```python
from build123d import *

# Parameters (mm, degrees)
SKETCH_1_W          = 25
SKETCH_1_H          = 8
SKETCH_1_R          = 1.2
EXTRUDE_2_DEPTH     = 4
SKETCH_2_W          = 10
SKETCH_2_H          = 0.8
EXTRUDE_3_DEPTH     = 0.8
SKETCH_3_W          = 7.5
SKETCH_3_H          = 8
SKETCH_3_R          = 1.2
EXTRUDE_4_DEPTH     = 1.5
SKETCH_4_W          = 25
SKETCH_4_H          = 1
CUT_EXTRUDE_1_DEPTH = 19.5


with BuildPart() as part:
    # 草图1 → 凸台-拉伸2 (new body)
    with BuildSketch(Plane.XY):
        with Locations((0.109785312, -0.548926558)):
            Rectangle(SKETCH_1_W, SKETCH_1_H)
        with Locations((-8.390214688, -2.048926558)):
            Circle(SKETCH_1_R, mode=Mode.SUBTRACT)
        with Locations((8.609785312, -2.048926558)):
            Circle(SKETCH_1_R, mode=Mode.SUBTRACT)
    extrude(amount=EXTRUDE_2_DEPTH)

    # 草图2 → 凸台-拉伸3 (add)
    with BuildSketch(Plane.XY.offset(4)):
        with Locations((0.109785312, -3.748926558)):
            Rectangle(SKETCH_2_W, SKETCH_2_H)
        with Locations((0.109785312, -2.148926558)):
            Rectangle(SKETCH_2_W, SKETCH_2_H)
        with Locations((0.109785312, -0.548926558)):
            Rectangle(SKETCH_2_W, SKETCH_2_H)
        with Locations((0.109785312, 2.651073442)):
            Rectangle(SKETCH_2_W, SKETCH_2_H)
        with Locations((0.109785312, 1.051073442)):
            Rectangle(SKETCH_2_W, SKETCH_2_H)
    extrude(amount=EXTRUDE_3_DEPTH)

    # 草图3 → 凸台-拉伸4 (add)
    # profile 1 of 2: a face of its own
    with BuildSketch(Plane.XY.offset(4)):
        with Locations((-8.640214688, -0.548926558)):
            Rectangle(SKETCH_3_W, SKETCH_3_H)
        with Locations((-8.390214688, -2.048926558)):
            Circle(SKETCH_3_R, mode=Mode.SUBTRACT)
    # profile 2 of 2: a face of its own
    with BuildSketch(Plane.XY.offset(4)):
        with Locations((8.859785312, -0.548926558)):
            Rectangle(SKETCH_3_W, SKETCH_3_H)
        with Locations((8.609785312, -2.048926558)):
            Circle(SKETCH_3_R, mode=Mode.SUBTRACT)
    extrude(amount=EXTRUDE_4_DEPTH)

    # 草图4 → 切除-拉伸1 (cut)
    with BuildSketch(Plane(origin=(0, 3.451073442, 0), x_dir=(1, 0, 0), z_dir=(0, 1, 0))):
        with Locations((0.109785312, -0.5)):
            Rectangle(SKETCH_4_W, SKETCH_4_H)
    extrude(amount=-CUT_EXTRUDE_1_DEPTH, mode=Mode.SUBTRACT)


solid = part.part
```
CAD build for the part. Positions are in the model's coordinates, mm. A direction names the side the tool comes from. Round coordinates to 2 decimals unless told otherwise and drop trailing zeros. Order: outer loops, then holes, each group sorted by start corner. A loop starts at its lowest first (then second) coordinate and runs counter-clockwise, first axis right, second up. Notation, with made-up numbers: (66, 33) - (93, 33) arc R21 ccw to (93, 39) - close; hole circle Ø1 at (45, 3.5). An arc over 180 degrees is marked (long way). Answer in a Markdown table with one row per item. Add a question column.
(1) Mould opens along Y. For faces 1 (the face through (0, -3, 4)), 2 (the face through (0, 3.451, 3)), 3 (the face through (0, 1, 4.8)) say: +Y half, -Y half, draft (parallel to the pull), parting line (faces both ways), or undercut.
(2) Band-saw the part on B-B on x = -1.5. List the corners of the cut face in (y, z).
(3) Band-saw the part on A-A on z = 5.2. List the corners of the cut face in (x, y).
(4) Band-saw the part on C-C on y = -1.5. List the corners of the cut face in (x, z).
(5) Drop flat-ended pins along their axis: pin 1 Ø0.9 at (x, z) = (-0.5, 4.5) entering from -Y; pin 2 Ø0.6 at (x, y) = (1, -3) entering from +Z; pin 3 Ø0.9 at (x, z) = (-1, 4.5) entering from +Y. Give the stop position or say it passes through.
(6) Band-saw the part on D-D on x = -8.75. List the corners of the cut face in (y, z).
(7) 3-axis set-ups, long thin cutter, end or side, ignore diameter. For faces 4 (the face through (0, 0.3, 4)), 5 (the face through (0, -3.7, 4.8)), 6 (the face through (12.61, -1, 3)): which of +Z, -Z, +X, -X, +Y, -Y reach the whole face in a straight line?
(8) Probe L1, parallel to X at y = 1.5, z = 4.7; L2, parallel to Z at x = 4.5, y = -1; L3, parallel to X at y = -1, z = 3.75. List the from-to ranges inside material, lowest first. Write a range as [from, to].
Data:
| question | item | result |
|---|---|---|
| 1 | face 1 | undercut |
| 1 | face 2 | +Y half |
| 1 | face 3 | draft |
| 2 | outline | (-4.55, 1) - (3.45, 1) - (3.45, 4) - (3.05, 4) - (3.05, 4.8) - (2.25, 4.8) - (2.25, 4) - (1.45, 4) - (1.45, 4.8) - (0.65, 4.8) - (0.65, 4) - (-0.15, 4) - (-0.15, 4.8) - (-0.95, 4.8) - (-0.95, 4) - (-1.75, 4) - (-1.75, 4.8) - (-2.55, 4.8) - (-2.55, 4) - (-3.35, 4) - (-3.35, 4.8) - (-4.15, 4.8) - (-4.15, 4) - (-4.55, 4) - close |
| 3 | outline | (-12.39, -4.55) - (-4.89, -4.55) - (-4.89, 3.45) - (-12.39, 3.45) - close; (5.11, -4.55) - (12.61, -4.55) - (12.61, 3.45) - (5.11, 3.45) - close; hole circle Ø2.4 at (-8.39, -2.05); hole circle Ø2.4 at (8.61, -2.05) |
| 4 | outline | (-12.39, 1) - (-9.46, 1) - (-9.46, 5.5) - (-12.39, 5.5) - close; (-7.32, 1) - (7.54, 1) - (7.54, 5.5) - (5.11, 5.5) - (5.11, 4) - (-4.89, 4) - (-4.89, 5.5) - (-7.32, 5.5) - close; (9.68, 1) - (12.61, 1) - (12.61, 5.5) - (9.68, 5.5) - close |
| 5 | pin 1 | stops at y = -4.15 |
| 5 | pin 2 | stops at z = 4 |
| 5 | pin 3 | stops at y = 3.05 |
| 6 | outline | (-4.55, 1) - (-3.19, 1) - (-3.19, 5.5) - (-4.55, 5.5) - close; (-0.9, 1) - (3.45, 1) - (3.45, 5.5) - (-0.9, 5.5) - close |
| 7 | face 4 | +Z |
| 7 | face 5 | +Z, +Y, -Y |
| 7 | face 6 | +Z, -Z, +X, +Y, -Y |
| 8 | L1 | x = [-12.39, -4.89], [5.11, 12.61] |
| 8 | L2 | z = [1, 4] |
| 8 | L3 | x = [-12.39, -8.97], [-7.81, 8.03], [9.19, 12.61] |
